Part model, mm, in its own coordinate system. Face numbers are marked on the shaded views. A direction names the side the tool comes from. Give positions to 0.01 mm unless a question says otherwise; leave off trailing zeros. Write each loop counter-clockwise with the first axis right and the second up, starting at its lowest first coordinate (ties: lowest second). Pieces come first, ordered by that corner, then holes. Notation, with made-up numbers: (10, 5.25) - (24, 5.25) arc R12 ccw to (24, 17.25) - close; hole circle Ø5 at (3.25, 71.25). An arc over 180 degrees is marked (long way). Answer in a Markdown table with one row per item. Add a question column.
1. Band-saw the part on A-A on x = 20. Write the cut outline in (y, z).
2. Pull direction Y, two halves, no side cores. Call the marked faces 1, 2 and 3: released by +Y, released by -Y, zero draft, split by the parting line, or undercut.
3. Band-saw the part on B-B on z = 5. Write the cut outline in (x, y).
4. Probe line 1 along Y through (x, z) = (28, 12); line 2 along X through (y, z) = (181, 4); line 3 along Y through (x, z) = (-21, 28). List the from-to ranges inside material, lowest first.
5. Which spindle directions (+Z, -Z, +X, -X, +Y, -Y) get a long thin tool onto all of the face, cutting with end or side? Do the marked faces 4, 5 and 6. Say none if no direction does.
6. Band-saw the part on D-D on z = 19. Write the cut outline in (x, y).
7. Drop flat-ended pins along their axis: pin 1 Ø24 at (x, y) = (-15.5, 60) entering from +Z; pin 2 Ø3 at (x, z) = (29.5, 28) entering from +Y; pin 3 Ø17.5 at (y, z) = (112.5, 11.5) entering from +X; pin 4 Ø8 at (x, y) = (-17.5, 106.5) entering from +Z. Give the stop position or say it passes through.
8. Band-saw the part on C-C on y = 114. Write the cut outline in (x, z).
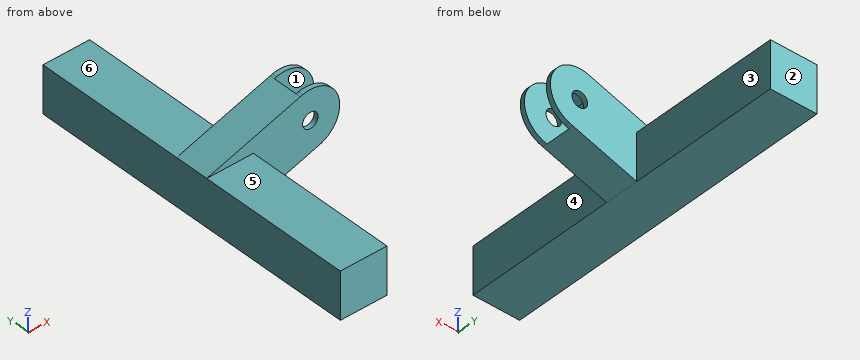
```python
from build123d import *

# Parameters (mm, degrees)
SKETCH1_W           = 30
SKETCH1_H           = 30
BOSS_EXTRUDE1_DEPTH = 217
SKETCH2_R           = 5
BOSS_EXTRUDE3_DEPTH = 119.5
SKETCH2_5_R         = 5
CUT_EXTRUDE1_DEPTH  = 116.5
SKETCH2_6_R         = 5
BOSS_EXTRUDE4_DEPTH = 100.5
SKETCH2_7_R         = 5
CUT_EXTRUDE2_DEPTH  = 97.5


with BuildPart() as part:
    # Sketch1 → Boss-Extrude1 (new body)
    with BuildSketch(Plane(origin=(0, 0, 0), x_dir=(1, 0, 0), z_dir=(0, 1, 0))):
        with Locations((-21.055045872, -9.729357798)):
            Rectangle(SKETCH1_W, SKETCH1_H)
    extrude(amount=BOSS_EXTRUDE1_DEPTH)

    # Sketch2 → Boss-Extrude3 (add)
    # profile 1 of 5: a face of its own
    with BuildSketch(Plane.XZ):
        with BuildLine():
            Line((24.087751056, 43.794339419), (-36.055045872, 24.729357798))
            Line((-36.055045872, 24.729357798), (-27.753478769, 24.729357798))
            Line((-27.753478769, 24.729357798), (16.642463995, 38.80266127))
            ThreePointArc((16.642463995, 38.80266127), (20.064375993, 41.747053421), (24.087751056, 43.794339419))
        make_face()
    # profile 2 of 5: a face of its own
    with BuildSketch(Plane.XZ):
        with BuildLine():
            Line((16.642463995, 38.80266127), (-27.753478769, 24.729357798))
            Line((-27.753478769, 24.729357798), (-6.055045872, 24.729357798))
            Line((-6.055045872, 24.729357798), (-6.055045872, -2.922177327))
            Line((-6.055045872, -2.922177327), (27.800199491, 7.411773197))
            ThreePointArc((27.800199491, 7.411773197), (12.793082951, 19.755992956), (16.642463995, 38.80266127))
        make_face()
    # profile 3 of 5: a face of its own
    with BuildSketch(Plane.XZ):
        with BuildLine():
            ThreePointArc((34.880858909, 7.705845626), (31.354459639, 7.223393087), (27.800199491, 7.411773197))
            Line((27.800199491, 7.411773197), (-6.055045872, -2.922177327))
            Line((-6.055045872, -2.922177327), (-6.055045872, -5.270642202))
            Line((-6.055045872, -5.270642202), (34.880858909, 7.705845626))
        make_face()
    # profile 4 of 5: a face of its own
    with BuildSketch(Plane.XZ):
        with BuildLine():
            Line((27.800199491, 7.411773197), (16.642463995, 38.80266127))
            ThreePointArc((16.642463995, 38.80266127), (12.793082951, 19.755992956), (27.800199491, 7.411773197))
        make_face()
    # profile 5 of 5: a face of its own
    with BuildSketch(Plane.XZ):
        with BuildLine():
            Line((25.663216571, 44.293754521), (24.087751056, 43.794339419))
            ThreePointArc((24.087751056, 43.794339419), (20.064375993, 41.747053421), (16.642463995, 38.80266127))
            Line((16.642463995, 38.80266127), (27.800199491, 7.411773197))
            ThreePointArc((27.800199491, 7.411773197), (31.354459639, 7.223393087), (34.880858909, 7.705845626))
            Line((34.880858909, 7.705845626), (37.631757216, 8.577867353))
            ThreePointArc((37.631757216, 8.577867353), (46.211503544, 15.520819013), (49.439613267, 26.07524616))
            ThreePointArc((49.439613267, 26.07524616), (49.213688832, 28.986343888), (48.541325909, 31.827727342))
            Line((48.541325909, 31.827727342), (47.968990161, 33.37819141))
            ThreePointArc((47.968990161, 33.37819141), (38.865020701, 43.022901823), (25.663216571, 44.293754521))
        make_face()
        with Locations(Location((30.57150852, 26.07524616, 0), (0, 0, 270))):
            Circle(SKETCH2_R, mode=Mode.SUBTRACT)
    extrude(amount=-BOSS_EXTRUDE3_DEPTH)

    # Sketch2_5 → Cut-Extrude1 (cut)
    # profile 1 of 3: a face of its own
    with BuildSketch(Plane.XZ):
        with BuildLine():
            Line((16.642463995, 38.80266127), (-27.753478769, 24.729357798))
            Line((-27.753478769, 24.729357798), (-6.055045872, 24.729357798))
            Line((-6.055045872, 24.729357798), (-6.055045872, -2.922177327))
            Line((-6.055045872, -2.922177327), (27.800199491, 7.411773197))
            ThreePointArc((27.800199491, 7.411773197), (12.793082951, 19.755992956), (16.642463995, 38.80266127))
        make_face()
    # profile 2 of 3: a face of its own
    with BuildSketch(Plane.XZ):
        with BuildLine():
            Line((27.800199491, 7.411773197), (16.642463995, 38.80266127))
            ThreePointArc((16.642463995, 38.80266127), (12.793082951, 19.755992956), (27.800199491, 7.411773197))
        make_face()
    # profile 3 of 3: a face of its own
    with BuildSketch(Plane.XZ):
        with BuildLine():
            Line((25.663216571, 44.293754521), (24.087751056, 43.794339419))
            ThreePointArc((24.087751056, 43.794339419), (20.064375993, 41.747053421), (16.642463995, 38.80266127))
            Line((16.642463995, 38.80266127), (27.800199491, 7.411773197))
            ThreePointArc((27.800199491, 7.411773197), (31.354459639, 7.223393087), (34.880858909, 7.705845626))
            Line((34.880858909, 7.705845626), (37.631757216, 8.577867353))
            ThreePointArc((37.631757216, 8.577867353), (46.211503544, 15.520819013), (49.439613267, 26.07524616))
            ThreePointArc((49.439613267, 26.07524616), (49.213688832, 28.986343888), (48.541325909, 31.827727342))
            Line((48.541325909, 31.827727342), (47.968990161, 33.37819141))
            ThreePointArc((47.968990161, 33.37819141), (38.865020701, 43.022901823), (25.663216571, 44.293754521))
        make_face()
        with Locations(Location((30.57150852, 26.07524616, 0), (0, 0, 270))):
            Circle(SKETCH2_5_R, mode=Mode.SUBTRACT)
    extrude(amount=-CUT_EXTRUDE1_DEPTH, mode=Mode.SUBTRACT)

    # Sketch2_6 → Boss-Extrude4 (add)
    # profile 1 of 3: a face of its own
    with BuildSketch(Plane.XZ):
        with BuildLine():
            Line((16.642463995, 38.80266127), (-27.753478769, 24.729357798))
            Line((-27.753478769, 24.729357798), (-6.055045872, 24.729357798))
            Line((-6.055045872, 24.729357798), (-6.055045872, -2.922177327))
            Line((-6.055045872, -2.922177327), (27.800199491, 7.411773197))
            ThreePointArc((27.800199491, 7.411773197), (12.793082951, 19.755992956), (16.642463995, 38.80266127))
        make_face()
    # profile 2 of 3: a face of its own
    with BuildSketch(Plane.XZ):
        with BuildLine():
            Line((27.800199491, 7.411773197), (16.642463995, 38.80266127))
            ThreePointArc((16.642463995, 38.80266127), (12.793082951, 19.755992956), (27.800199491, 7.411773197))
        make_face()
    # profile 3 of 3: a face of its own
    with BuildSketch(Plane.XZ):
        with BuildLine():
            Line((25.663216571, 44.293754521), (24.087751056, 43.794339419))
            ThreePointArc((24.087751056, 43.794339419), (20.064375993, 41.747053421), (16.642463995, 38.80266127))
            Line((16.642463995, 38.80266127), (27.800199491, 7.411773197))
            ThreePointArc((27.800199491, 7.411773197), (31.354459639, 7.223393087), (34.880858909, 7.705845626))
            Line((34.880858909, 7.705845626), (37.631757216, 8.577867353))
            ThreePointArc((37.631757216, 8.577867353), (46.211503544, 15.520819013), (49.439613267, 26.07524616))
            ThreePointArc((49.439613267, 26.07524616), (49.213688832, 28.986343888), (48.541325909, 31.827727342))
            Line((48.541325909, 31.827727342), (47.968990161, 33.37819141))
            ThreePointArc((47.968990161, 33.37819141), (38.865020701, 43.022901823), (25.663216571, 44.293754521))
        make_face()
        with Locations(Location((30.57150852, 26.07524616, 0), (0, 0, 270))):
            Circle(SKETCH2_6_R, mode=Mode.SUBTRACT)
    extrude(amount=-BOSS_EXTRUDE4_DEPTH)

    # Sketch2_7 → Cut-Extrude2 (cut)
    # profile 1 of 5: a face of its own
    with BuildSketch(Plane.XZ):
        with BuildLine():
            Line((25.663216571, 44.293754521), (24.087751056, 43.794339419))
            ThreePointArc((24.087751056, 43.794339419), (20.064375993, 41.747053421), (16.642463995, 38.80266127))
            Line((16.642463995, 38.80266127), (27.800199491, 7.411773197))
            ThreePointArc((27.800199491, 7.411773197), (31.354459639, 7.223393087), (34.880858909, 7.705845626))
            Line((34.880858909, 7.705845626), (37.631757216, 8.577867353))
            ThreePointArc((37.631757216, 8.577867353), (46.211503544, 15.520819013), (49.439613267, 26.07524616))
            ThreePointArc((49.439613267, 26.07524616), (49.213688832, 28.986343888), (48.541325909, 31.827727342))
            Line((48.541325909, 31.827727342), (47.968990161, 33.37819141))
            ThreePointArc((47.968990161, 33.37819141), (38.865020701, 43.022901823), (25.663216571, 44.293754521))
        make_face()
        with Locations(Location((30.57150852, 26.07524616, 0), (0, 0, 270))):
            Circle(SKETCH2_7_R, mode=Mode.SUBTRACT)
    # profile 2 of 5: a face of its own
    with BuildSketch(Plane.XZ):
        with BuildLine():
            Line((27.800199491, 7.411773197), (16.642463995, 38.80266127))
            ThreePointArc((16.642463995, 38.80266127), (12.793082951, 19.755992956), (27.800199491, 7.411773197))
        make_face()
    # profile 3 of 5: a face of its own
    with BuildSketch(Plane.XZ):
        with BuildLine():
            Line((16.642463995, 38.80266127), (-27.753478769, 24.729357798))
            Line((-27.753478769, 24.729357798), (-6.055045872, 24.729357798))
            Line((-6.055045872, 24.729357798), (-6.055045872, -2.922177327))
            Line((-6.055045872, -2.922177327), (27.800199491, 7.411773197))
            ThreePointArc((27.800199491, 7.411773197), (12.793082951, 19.755992956), (16.642463995, 38.80266127))
        make_face()
    # profile 4 of 5: a face of its own
    with BuildSketch(Plane.XZ):
        with BuildLine():
            Line((24.087751056, 43.794339419), (-36.055045872, 24.729357798))
            Line((-36.055045872, 24.729357798), (-27.753478769, 24.729357798))
            Line((-27.753478769, 24.729357798), (16.642463995, 38.80266127))
            ThreePointArc((16.642463995, 38.80266127), (20.064375993, 41.747053421), (24.087751056, 43.794339419))
        make_face()
    # profile 5 of 5: a face of its own
    with BuildSketch(Plane.XZ):
        with BuildLine():
            ThreePointArc((34.880858909, 7.705845626), (31.354459639, 7.223393087), (27.800199491, 7.411773197))
            Line((27.800199491, 7.411773197), (-6.055045872, -2.922177327))
            Line((-6.055045872, -2.922177327), (-6.055045872, -5.270642202))
            Line((-6.055045872, -5.270642202), (34.880858909, 7.705845626))
        make_face()
    extrude(amount=-CUT_EXTRUDE2_DEPTH, mode=Mode.SUBTRACT)


solid = part.part
```
Values:
| question | item | result |
|---|---|---|
| 1 | outline | (97.5, 2.99) - (119.5, 2.99) - (119.5, 42.5) - (97.5, 42.5) - close; hole (100.5, 5.03) - (116.5, 5.03) - (116.5, 41.7) - (100.5, 41.7) - close |
| 2 | face 1 | undercut |
| 2 | face 2 | released by +Y |
| 2 | face 3 | zero draft |
| 3 | outline | (-36.06, 0) - (-6.06, 0) - (-6.06, 97.5) - (26.34, 97.5) - (26.34, 119.5) - (-6.06, 119.5) - (-6.06, 217) - (-36.06, 217) - close; hole (-6.06, 100.5) - (19.9, 100.5) - (19.9, 116.5) - (-6.06, 116.5) - close |
| 4 | line 1 | y = 97.5 to 100.5, 116.5 to 119.5 |
| 4 | line 2 | x = -36.06 to -6.06 |
| 4 | line 3 | y = 97.5 to 119.5 |
| 5 | face 4 | +Z, -Z, +X, -Y |
| 5 | face 5 | +Z, +X, -X, -Y |
| 5 | face 6 | +Z, +X, -X, +Y |
| 6 | outline | (-36.06, 0) - (-6.06, 0) - (-6.06, 97.5) - (48.06, 97.5) - (48.06, 100.5) - (-6.06, 100.5) - (-6.06, 116.5) - (48.06, 116.5) - (48.06, 119.5) - (-6.06, 119.5) - (-6.06, 217) - (-36.06, 217) - close |
| 7 | pin 1 | stops at z = 24.73 |
| 7 | pin 2 | passes through |
| 7 | pin 3 | stops at x = 48.17 |
| 7 | pin 4 | stops at z = 31.88 |
| 8 | outline | (-36.06, -5.27) - (-6.06, -5.27) - (34.88, 7.71) arc R18.87 cw to (27.8, 7.41) - (-6.06, -2.92) - (-6.06, 24.73) - (-27.75, 24.73) - (16.64, 38.8) arc R18.87 cw to (24.09, 43.79) - (-36.06, 24.73) - close |
